The listing builds one solid part. Answer for the finished solid, in the listing's coordinates (mm). Face numbers are marked on the shaded views. A direction names the side the tool comes from. Give positions to 0.01 mm unless a question says otherwise; leave off trailing zeros. Write each loop counter-clockwise with the first axis right and the second up, starting at its lowest first coordinate (ties: lowest second). Pieces come first, ordered by that corner, then holes. Notation, with made-up numbers: (76, -27.5) -> (134, -27.5) arc R11 ccw to (134, -13.5) -> close; hole circle Ø8 at (77.5, 70.25). An arc over 180 degrees is marked (long way). Put each result on its own line as item: value. Start each with the question number.
1) Flat-ended cylindrical pins translate along their axes: pin 1 Ø3.5 at (x, y) = (-0.5, 8.5) entering from -Z; pin 2 Ø12 at (x, y) = (-1.5, 6.5) entering from +Z; pin 3 Ø8 at (x, y) = (-14.5, 11) entering from -Z. Find the tip coordinate at first contact, or state that the pin passes through.
2) Find the intervals of material crossed by line 1 along Z through (x, y) = (7, 10.5); line 2 along Z through (x, y) = (-6.5, 18); line 3 along X through (y, z) = (2, 0.5), in increasing order. Write a range as from..to.
3) For a pull along Z with two mould halves and no side action, classify the marked faces 1, 2 and 3 as released by +Z, released by -Z, zero draft, split by the parting line, or undercut.
4) A cutting plane is placed at B-B (y = 13.75). Write down the section's boundary in (x, z), then the cut area to 3 significant figures.
5) A cutting plane is placed at C-C (z = 2). Write down the section's boundary in (x, y), then the cut area to 3 significant figures.
6) A cutting plane is placed at A-A (x = 0). Write down the section's boundary in (y, z).
7) For the marked faces 4, 5 and 6, determine the directions among +Z, -Z, +X, -X, +Y, -Y from which every point of the face is accessible in a straight line to the end or side of a thin tool.
8) A cutting plane is placed at D-D (x = -6.5). Write down the section's boundary in (y, z).
from build123d import *

# Parameters (mm, degrees)
SKETCH1_R           = 17.5
BOSS_EXTRUDE1_DEPTH = 20
SKETCH2_R           = 21.5
BOSS_EXTRUDE2_DEPTH = 3
SKETCH3_W           = 19
SKETCH3_H           = 8.5
CUT_EXTRUDE3_DEPTH  = 23
FILLET11_R          = 4
FILLET12_R          = 4
BOSS_EXTRUDE4_START = -3
SKETCH6_R           = 22.520770935
SKETCH6_R_2         = 21.5
BOSS_EXTRUDE4_DEPTH = 3


with BuildPart() as part:
    # Sketch1 → Boss-Extrude1 (new body)
    with BuildSketch(Plane(origin=(0, 0, 0), x_dir=(1, 0, 0), z_dir=(0, 1, 0))):
        with Locations(Location((0, 0, 0), (0, 0, 270))):
            Circle(SKETCH1_R)
    extrude(amount=BOSS_EXTRUDE1_DEPTH)

    # Sketch2 → Boss-Extrude2 (add)
    with BuildSketch(Plane(origin=(0, 20, 0), x_dir=(1, 0, 0), z_dir=(0, 1, 0))):
        with Locations(Location((0, 0, 0), (0, 0, 270))):
            Circle(SKETCH2_R)
    extrude(amount=BOSS_EXTRUDE2_DEPTH)

    # Sketch3 → Cut-Extrude3 (cut)
    with BuildSketch(Plane(origin=(0, 23, 0), x_dir=(1, 0, 0), z_dir=(0, 1, 0))):
        with Locations((0, 0.083811037)):
            Rectangle(SKETCH3_W, SKETCH3_H)
        with Locations((0, 10.083811037)):
            Rectangle(SKETCH3_W, SKETCH3_H)
        with Locations((0, -9.916188963)):
            Rectangle(SKETCH3_W, SKETCH3_H)
    extrude(amount=-CUT_EXTRUDE3_DEPTH, mode=Mode.SUBTRACT)

    # Fillet11
    fillet11_edges = [part.edges().sort_by_distance(p)[0] for p in [
        (9.5, 11.5, 4.166188963),
        (-9.5, 11.5, 4.166188963),
        (-9.5, 11.5, -4.333811037),
        (9.5, 11.5, -4.333811037),
        (9.5, 11.5, 14.166188963),
        (-9.5, 11.5, 14.166188963),
        (-9.5, 11.5, 5.666188963),
        (9.5, 11.5, 5.666188963),
    ]]
    fillet(fillet11_edges, radius=FILLET11_R)

    # Fillet12
    fillet12_edges = [part.edges().sort_by_distance(p)[0] for p in [
        (9.5, 11.5, -14.333811037),
        (9.5, 11.5, -5.833811037),
        (-9.5, 11.5, -5.833811037),
        (-9.5, 11.5, -14.333811037),
    ]]
    fillet(fillet12_edges, radius=FILLET12_R)

    # Sketch6 → Boss-Extrude4 (add)
    with BuildSketch(Plane(origin=(0, 23, 0), x_dir=(1, 0, 0), z_dir=(0, 1, 0)).offset(BOSS_EXTRUDE4_START)):
        with Locations(Location((0, 0, 0), (0, 0, 270))):
            Circle(SKETCH6_R)
        Circle(SKETCH6_R_2, mode=Mode.SUBTRACT)
    extrude(amount=BOSS_EXTRUDE4_DEPTH)


solid = part.part
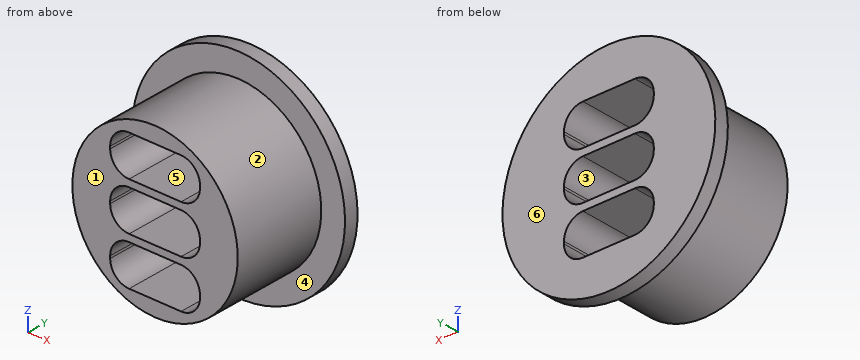
Reply:
1. pin 1: stops at z = -17.5
1. pin 2: stops at z = 17.5
1. pin 3: stops at z = -14
2. line 1: z = -16.04..-14.04, -6.13..-4.04, 3.87..5.96, 13.87..16.04
2. line 2: z = -16.25..-14.21, -5.96..-4.21, 4.04..5.79, 14.04..16.25
2. line 3: x = -17.49..-9.49, 9.49..17.49
3. face 1: zero draft
3. face 2: split by the parting line
3. face 3: undercut
4. outline: circle Ø35 at (0, 0); hole (-9.5, -10.33) arc R4 ccw to (-5.5, -14.33) -> (5.5, -14.33) arc R4 ccw to (9.5, -10.33) -> (9.5, -9.83) arc R4 ccw to (5.5, -5.83) -> (-5.5, -5.83) arc R4 ccw to (-9.5, -9.83) -> close; hole (-9.5, -0.33) arc R4 ccw to (-5.5, -4.33) -> (5.5, -4.33) arc R4 ccw to (9.5, -0.33) -> (9.5, 0.17) arc R4 ccw to (5.5, 4.17) -> (-5.5, 4.17) arc R4 ccw to (-9.5, 0.17) -> close; hole (-9.5, 9.67) arc R4 ccw to (-5.5, 5.67) -> (5.5, 5.67) arc R4 ccw to (9.5, 9.67) -> (9.5, 10.17) arc R4 ccw to (5.5, 14.17) -> (-5.5, 14.17) arc R4 ccw to (-9.5, 10.17) -> close
4. area: 519 mm2
5. outline: (-22.43, 20) -> (-17.39, 20) -> (-17.39, 0) -> (-9.05, 0) -> (-9.05, 23) -> (-22.43, 23) -> close; (9.05, 0) -> (17.39, 0) -> (17.39, 20) -> (22.43, 20) -> (22.43, 23) -> (9.05, 23) -> close
5. area: 413 mm2
6. outline: (0, -17.5) -> (20, -17.5) -> (20, -22.52) -> (23, -22.52) -> (23, -14.33) -> (0, -14.33) -> close; (0, -5.83) -> (23, -5.83) -> (23, -4.33) -> (0, -4.33) -> close; (0, 4.17) -> (23, 4.17) -> (23, 5.67) -> (0, 5.67) -> close; (0, 14.17) -> (23, 14.17) -> (23, 22.52) -> (20, 22.52) -> (20, 17.5) -> (0, 17.5) -> close
7. face 4: -Y
7. face 5: +Y, -Y
7. face 6: +Z, -Z, +X, -X, +Y
8. outline: (0, -16.25) -> (20, -16.25) -> (20, -21.56) -> (23, -21.56) -> (23, -14.21) -> (0, -14.21) -> close; (0, -5.96) -> (23, -5.96) -> (23, -4.21) -> (0, -4.21) -> close; (0, 4.04) -> (23, 4.04) -> (23, 5.79) -> (0, 5.79) -> close; (0, 14.04) -> (23, 14.04) -> (23, 21.56) -> (20, 21.56) -> (20, 16.25) -> (0, 16.25) -> close
